The figure shows three views and two pictorial views of one solid part (mm, origin at its lowest corner). Answer the questions. Coordinates: 2 decimals unless noted, no trailing zeros. Order: outer loops, then holes, each group sorted by start corner. A loop starts at its lowest first (then second) coordinate and runs counter-clockwise, first axis right, second up. Notation, with made-up numbers: (57, -13.5) -> (88, -13.5) arc R25 cw to (88, 22.5) -> close; hole circle Ø3 at (80.25, 51.5). An arc over 180 degrees is marked (long way). Return JSON: item names as keys, results as strings. Group by question number.
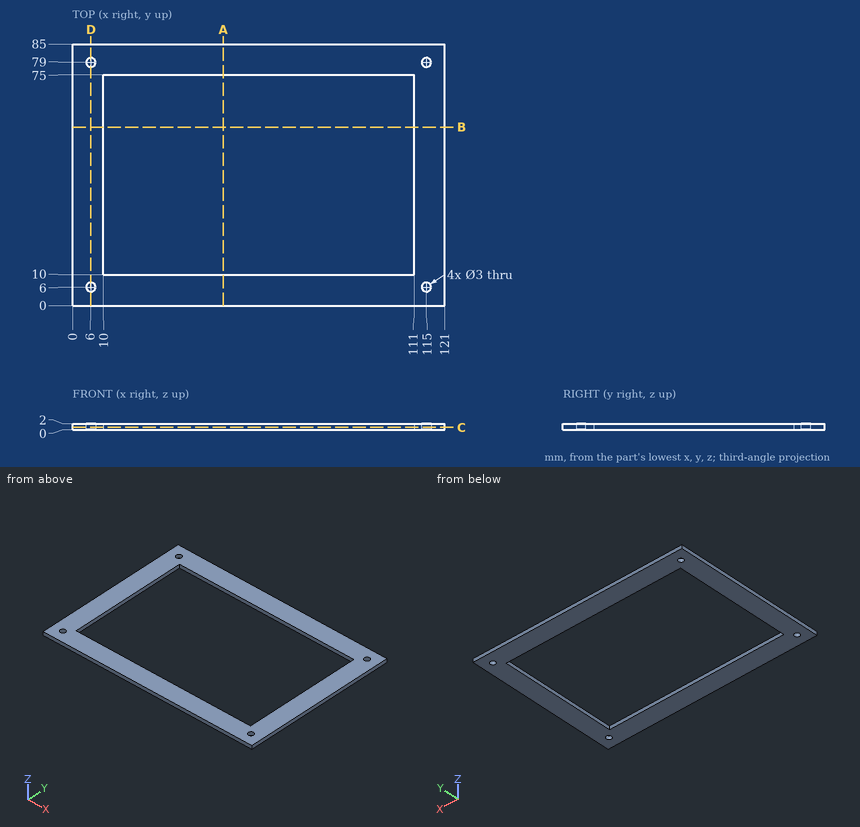
1. Find section B-B on y = 58. Determine the outline of the cut face in (x, z), and give its area (3 significant figures).
2. Given pin 1 (2.5 mm diameter, centred on x = 115, y = 79, fed in from +Z) (1 decimal); pin 2 (2 mm diameter, centred on x = 96, y = 10.5, fed in from +Z), each flat-ended and moving along its own axis, determine where each tip first touches the part or whether it passes through.
3. Find section C-C on z = 0.75. Determine the outline of the cut face in (x, y), and give its area (3 significant figures).
4. Straight lines are drawn through the part: L1, parallel to Y at x = 115, z = 1.2; L2, parallel to X at y = 79, z = 1.45; L3, parallel to Y at x = 19.5, z = 1.9. For each, find the intervals that lie inside material, in ascending order.
5. Find section A-A on x = 49. Determine the outline of the cut face in (y, z).
6. Find section D-D on x = 6. Determine the outline of the cut face in (y, z), and give its area (3 significant figures).
Result:
{
 "1": {"outline": "(0, 0) -> (10, 0) -> (10, 2) -> (0, 2) -> close; (111, 0) -> (121, 0) -> (121, 2) -> (111, 2) -> close", "area": "40.0 mm^2"},
 "2": {"pin 1": "through", "pin 2": "z = 2"},
 "3": {"outline": "(0, 0) -> (121, 0) -> (121, 85) -> (0, 85) -> close; hole circle Ø3 at (6, 6); hole circle Ø3 at (6, 79); hole (10, 10) -> (111, 10) -> (111, 75) -> (10, 75) -> close; hole circle Ø3 at (115, 6); hole circle Ø3 at (115, 79)", "area": "3,690 mm^2"},
 "4": {"L1": "0 to 4.5, 7.5 to 77.5, 80.5 to 85", "L2": "0 to 4.5, 7.5 to 113.5, 116.5 to 121", "L3": "0 to 10, 75 to 85"},
 "5": {"outline": "(0, 0) -> (10, 0) -> (10, 2) -> (0, 2) -> close; (75, 0) -> (85, 0) -> (85, 2) -> (75, 2) -> close"},
 "6": {"outline": "(0, 0) -> (4.5, 0) -> (4.5, 2) -> (0, 2) -> close; (7.5, 0) -> (77.5, 0) -> (77.5, 2) -> (7.5, 2) -> close; (80.5, 0) -> (85, 0) -> (85, 2) -> (80.5, 2) -> close", "area": "158 mm^2"}
}
